```python
from build123d import *

# Parameters (mm, degrees)
SKETCH1_W               = 192.857142858
SKETCH1_H               = 177.8
BOSS_EXTRUDE1_DEPTH     = 16
SKETCH3_R               = 6.25
CUT_EXTRUDE1_DEPTH      = 12.7
CUT_EXTRUDE2_DEPTH      = 133.12751185
CUT_EXTRUDE2_DEPTH_BACK = 133.12751185
SKETCH6_R               = 3.5
CUT_EXTRUDE3_DEPTH      = 133.12751185
CUT_EXTRUDE3_DEPTH_BACK = 133.12751185
SKETCH7_W               = 15.5
SKETCH7_H               = 15.2
SKETCH17_W              = 58.35
SKETCH17_H              = 177.8
CUT_EXTRUDE10_DEPTH     = 133.12751185
SKETCH18_W              = 17
SKETCH18_H              = 10
CUT_EXTRUDE11_DEPTH     = 99.419229548
FILLET1_R               = 2
SKETCH19_W              = 48
SKETCH19_H              = 10
BOSS_EXTRUDE2_DEPTH     = 18
SKETCH20_W              = 177.8
SKETCH20_H              = 16
BOSS_EXTRUDE3_DEPTH     = 35
SKETCH21_W              = 10
SKETCH21_H              = 107
BOSS_EXTRUDE4_DEPTH     = 18
SKETCH23_W              = 17
SKETCH23_H              = 10
CUT_EXTRUDE12_DEPTH     = 30
FILLET2_R               = 2
SKETCH22_W              = 19.5
SKETCH22_H              = 150
CUT_EXTRUDE13_DEPTH     = 1
SKETCH24_W              = 29.328571429
SKETCH24_H              = 10
BOSS_EXTRUDE5_DEPTH     = 18


with BuildPart() as part:
    # Sketch1 → Boss-Extrude1 (new body)
    with BuildSketch(Plane(origin=(0, 0, 0), x_dir=(1, 0, 0), z_dir=(0, 1, 0))):
        Rectangle(SKETCH1_W, SKETCH1_H)
    extrude(amount=BOSS_EXTRUDE1_DEPTH)

    # Sketch3 → Cut-Extrude1 (cut)
    with BuildSketch(Plane(origin=(0, 16, 0), x_dir=(1, 0, 0), z_dir=(0, 1, 0))):
        with Locations(Location((-25.4, 76.2, 0), (0, 0, 270))):
            Circle(SKETCH3_R)
        with Locations(Location((25.4, 76.2, 0), (0, 0, 270))):
            Circle(SKETCH3_R)
        with Locations(Location((25.4, -76.2, 0), (0, 0, 90))):
            Circle(SKETCH3_R)
        with Locations(Location((-25.4, -76.2, 0), (0, 0, 90))):
            Circle(SKETCH3_R)
    extrude(amount=-CUT_EXTRUDE1_DEPTH, mode=Mode.SUBTRACT)

    # Sketch6 → Cut-Extrude2 (cut, two sides: drawn at the far end of the back side and taken through both)
    with BuildSketch(Plane(origin=(0, 0, 0), x_dir=(-1, 0, 0), z_dir=(0, -1, 0)).offset(-CUT_EXTRUDE2_DEPTH_BACK)):
        with Locations(Location((25.4, -76.2, 0), (0, 0, 90))):
            Circle(SKETCH6_R)
        with Locations(Location((-25.4, -76.2, 0), (0, 0, 90))):
            Circle(SKETCH6_R)
        with Locations(Location((-25.4, 76.2, 0), (0, 0, 270))):
            Circle(SKETCH6_R)
        with Locations(Location((25.4, 76.2, 0), (0, 0, 270))):
            Circle(SKETCH6_R)
    extrude(amount=CUT_EXTRUDE2_DEPTH + CUT_EXTRUDE2_DEPTH_BACK, mode=Mode.SUBTRACT)

    # Sketch7 → Cut-Extrude3 (cut, two sides: drawn at the far end of the back side and taken through both)
    with BuildSketch(Plane(origin=(0, 16, 0), x_dir=(1, 0, 0), z_dir=(0, 1, 0)).offset(-CUT_EXTRUDE3_DEPTH_BACK)):
        Rectangle(SKETCH7_W, SKETCH7_H)
    extrude(amount=CUT_EXTRUDE3_DEPTH + CUT_EXTRUDE3_DEPTH_BACK, mode=Mode.SUBTRACT)

    # Sketch17 → Cut-Extrude10 (cut, symmetric)
    with BuildSketch(Plane(origin=(0, 16, 0), x_dir=(1, 0, 0), z_dir=(0, 1, 0))):
        with Locations((67.253571429, 0)):
            Rectangle(SKETCH17_W, SKETCH17_H)
    cut_extrude10 = extrude(amount=CUT_EXTRUDE10_DEPTH, both=True, mode=Mode.SUBTRACT)

    # Mirror5: Cut-Extrude10 across plane
    add(cut_extrude10.mirror(Plane(origin=(-0.5, 0, 0), x_dir=(0, 0, 1), z_dir=(1, 0, 0))), mode=Mode.SUBTRACT)

    # Sketch18 → Cut-Extrude11 (cut, through all)
    with BuildSketch(Plane(origin=(0, 16, 0), x_dir=(1, 0, 0), z_dir=(0, 1, 0))):
        with Locations((0, -73.9)):
            Rectangle(SKETCH18_W, SKETCH18_H)
    extrude(amount=-CUT_EXTRUDE11_DEPTH, mode=Mode.SUBTRACT)

    # Fillet1
    fillet1_edges = [part.edges().sort_by_distance(p)[0] for p in [
        (-8.5, 8, 78.9),
        (-8.5, 8, 68.9),
        (8.5, 8, 68.9),
        (8.5, 8, 78.9),
    ]]
    fillet(fillet1_edges, radius=FILLET1_R)

    # Sketch19 → Boss-Extrude2 (add)
    with BuildSketch(Plane(origin=(0, 16, 0), x_dir=(1, 0, 0), z_dir=(0, 1, 0))):
        with Locations((33.921428571, 34.6)):
            Rectangle(SKETCH19_W, SKETCH19_H)
    extrude(amount=BOSS_EXTRUDE2_DEPTH)

    # Sketch20 → Boss-Extrude3 (add)
    with BuildSketch(Plane(origin=(38.078571429, 0, 0), x_dir=(0, 0, -1), z_dir=(1, 0, 0))):
        with Locations((0, 8)):
            Rectangle(SKETCH20_W, SKETCH20_H)
    extrude(amount=BOSS_EXTRUDE3_DEPTH)

    # Sketch21 → Boss-Extrude4 (add)
    with BuildSketch(Plane(origin=(0, 16, 0), x_dir=(1, 0, 0), z_dir=(0, 1, 0))):
        with Locations((62.921428571, -13.75)):
            Rectangle(SKETCH21_W, SKETCH21_H)
    extrude(amount=BOSS_EXTRUDE4_DEPTH)

    # Sketch23 → Cut-Extrude12 (cut)
    with BuildSketch(Plane(origin=(0, 16, 0), x_dir=(1, 0, 0), z_dir=(0, 1, 0))):
        with Locations((0, 73.9)):
            Rectangle(SKETCH23_W, SKETCH23_H)
    extrude(amount=-CUT_EXTRUDE12_DEPTH, mode=Mode.SUBTRACT)

    # Fillet2
    fillet2_edges = [part.edges().sort_by_distance(p)[0] for p in [
        (-8.5, 8, -68.9),
        (-8.5, 8, -78.9),
        (8.5, 8, -78.9),
        (8.5, 8, -68.9),
    ]]
    fillet(fillet2_edges, radius=FILLET2_R)

    # Sketch22 → Cut-Extrude13 (cut)
    with BuildSketch(Plane(origin=(0, 16, 0), x_dir=(1, 0, 0), z_dir=(0, 1, 0))):
        with Locations((0, 0.096227078)):
            Rectangle(SKETCH22_W, SKETCH22_H)
    extrude(amount=-CUT_EXTRUDE13_DEPTH, mode=Mode.SUBTRACT)

    # Sketch24 → Boss-Extrude5 (add)
    with BuildSketch(Plane(origin=(0, 16, 0), x_dir=(1, 0, 0), z_dir=(0, 1, 0))):
        with Locations((-24.414285715, 34.6)):
            Rectangle(SKETCH24_W, SKETCH24_H)
    extrude(amount=BOSS_EXTRUDE5_DEPTH)


solid = part.part
```
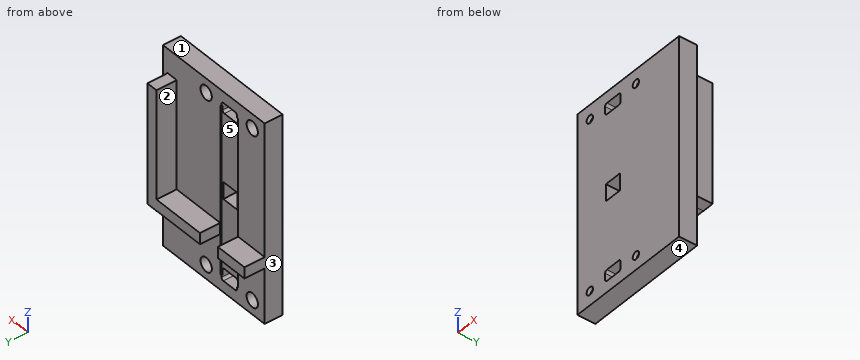
Design review of the part built by this model. Coordinates are the model's own, in mm. Face numbers are marked on the shaded views. A direction names the side the tool comes from. Give positions to 0.01 mm unless a question says otherwise; leave off trailing zeros. Write each loop counter-clockwise with the first axis right and the second up, starting at its lowest first coordinate (ties: lowest second). Pieces come first, ordered by that corner, then holes. Notation, with made-up numbers: (67, -32) -> (125, -32) arc R9 cw to (125, -24) -> close; hole circle Ø10 at (66.5, -12). An arc over 180 degrees is marked (long way). Answer in a Markdown table with one row per item.
(1) Consider section C-C (z = 4.5). State the section outline as (x, y) points.
Results:
| item | result |
|---|---|
| outline | (-39.08, 0) -> (-7.75, 0) -> (-7.75, 15) -> (-9.75, 15) -> (-9.75, 16) -> (-39.08, 16) -> close; (7.75, 0) -> (73.08, 0) -> (73.08, 16) -> (67.92, 16) -> (67.92, 34) -> (57.92, 34) -> (57.92, 16) -> (9.75, 16) -> (9.75, 15) -> (7.75, 15) -> close |
(2) Consider section A-A (y = 20.5). State the section outline as (x, z) points, then the cut area to 3 significant figures.
Results:
| item | result |
|---|---|
| outline | (-39.08, -39.6) -> (-9.75, -39.6) -> (-9.75, -29.6) -> (-39.08, -29.6) -> close; (9.92, -39.6) -> (57.92, -39.6) -> (57.92, -39.75) -> (67.92, -39.75) -> (67.92, 67.25) -> (57.92, 67.25) -> (57.92, -29.6) -> (9.92, -29.6) -> close |
| area | 1,840 mm2 |
(3) To check wall thickness, follow probe 1 along X at (y, z) = (1.6, -76.2); probe 2 along X at (y, z) = (7, 80); probe 3 along Y at (x, z) = (5.5, -31). State the ranges of each line that lie inside material, in increasing order.
Results:
| item | result |
|---|---|
| probe 1 | -39.08 to -28.9, -21.9 to -8.5, 8.5 to 21.9, 28.9 to 73.08 |
| probe 2 | -39.08 to -30.36, -20.44 to 20.44, 30.36 to 73.08 |
| probe 3 | 0 to 15 |
(4) Consider section B-B (y = 6). State the section outline as (x, z) points, then the cut area to 3 significant figures.
Results:
| item | result |
|---|---|
| outline | (-39.08, -88.9) -> (73.08, -88.9) -> (73.08, 88.9) -> (-39.08, 88.9) -> close; hole circle Ø12.5 at (-25.4, -76.2); hole circle Ø12.5 at (-25.4, 76.2); hole (-8.5, -76.9) arc R2 ccw to (-6.5, -78.9) -> (6.5, -78.9) arc R2 ccw to (8.5, -76.9) -> (8.5, -70.9) arc R2 ccw to (6.5, -68.9) -> (-6.5, -68.9) arc R2 ccw to (-8.5, -70.9) -> close; hole (-8.5, 70.9) arc R2 ccw to (-6.5, 68.9) -> (6.5, 68.9) arc R2 ccw to (8.5, 70.9) -> (8.5, 76.9) arc R2 ccw to (6.5, 78.9) -> (-6.5, 78.9) arc R2 ccw to (-8.5, 76.9) -> close; hole (-7.75, -7.6) -> (7.75, -7.6) -> (7.75, 7.6) -> (-7.75, 7.6) -> close; hole circle Ø12.5 at (25.4, -76.2); hole circle Ø12.5 at (25.4, 76.2) |
| area | 18,900 mm2 |
(5) For the marked faces 1 and 2, list the 3-axis set-ups (+Z, -Z, +X, -X, +Y, -Y) from which the entire face can be reached by the end or side of a thin tool; tool diameter is ignored.
Results:
| item | result |
|---|---|
| face 1 | +Z, +X, -X, +Y, -Y |
| face 2 | +Z, -X, +Y |
(6) Consider section D-D (x = -25.4). State the section outline as (y, z) points, then the cut area to 3 significant figures.
Results:
| item | result |
|---|---|
| outline | (0, -88.9) -> (16, -88.9) -> (16, -82.45) -> (3.3, -82.45) -> (3.3, -79.7) -> (0, -79.7) -> close; (0, -72.7) -> (3.3, -72.7) -> (3.3, -69.95) -> (16, -69.95) -> (16, -39.6) -> (34, -39.6) -> (34, -29.6) -> (16, -29.6) -> (16, 69.95) -> (3.3, 69.95) -> (3.3, 72.7) -> (0, 72.7) -> close; (0, 79.7) -> (3.3, 79.7) -> (3.3, 82.45) -> (16, 82.45) -> (16, 88.9) -> (0, 88.9) -> close |
| area | 2,660 mm2 |
(7) Mouldability with a two-part tool opening along X and no side actions: class the marked faces 3, 4 and 5 as +X half, -X half, draft (parallel to the pull), parting line (faces both ways), or undercut.
Results:
| item | result |
|---|---|
| face 3 | -X half |
| face 4 | draft |
| face 5 | undercut |
(8) Clearance check with flat-ended pins moving along their axes: pin 1 (4 mm diameter, centred on x = 51, z = -24.5, fed in from +Y); pin 2 (5.5 mm diameter, centred on x = -25.4, z = -76.2, fed in from -Y); pin 3 (4 mm diameter, centred on x = -12, y = 21, fed in from +Z); pin 4 (1.5 mm diameter, centred on y = 24.5, z = 6.5, fed in from -X). State where each tip first meets the part, or that it passes through.
Results:
| item | result |
|---|---|
| pin 1 | y = 16 |
| pin 2 | through |
| pin 3 | z = -29.6 |
| pin 4 | x = 57.92 |
